Geometry check sheet. Reference: the model listing, model coordinates, mm. Face numbers are marked on the shaded views. A direction names the side the tool comes from. Coordinates: 2 decimals unless noted, no trailing zeros. Loops run counter-clockwise (first coordinate to the right, second up) from the corner with the lowest first, then second, coordinate; pieces in that order, holes last. Notation, with made-up numbers: (4.25, 15.5) -> (45.25, 15.5) arc R26 cw to (45.25, 50.5) -> close; hole circle Ø4 at (-33.5, 30). An arc over 180 degrees is marked (long way). Answer as a JSON object with one key per item and string values.
from build123d import *

# Parameters (mm, degrees)
F0_W     = 334.264
F0_H     = 232.664
F0_W_2   = 330.2
F0_H_2   = 228.6
F1_DEPTH = 53.34
F2_DEPTH = 1.27
F3_W     = 360.172
F3_H     = 258.572
F3_W_2   = 334.264
F3_H_2   = 232.664
F4_DEPTH = 2.032
F5_R     = 5.08
F6_R     = 3.175
F7_DEPTH = 1.271


with BuildPart() as f1:
    # F0 (on Top) → F1 (new body)
    with BuildSketch(Plane.XY):
        with Locations((167.132, 116.332)):
            Rectangle(F0_W, F0_H)
        with Locations((167.132, 116.332)):
            Rectangle(F0_W_2, F0_H_2, mode=Mode.SUBTRACT)
    extrude(amount=F1_DEPTH)

    # F0 (on Top) → F2 (join)
    with BuildSketch(Plane.XY):
        with Locations((167.132, 116.332)):
            Rectangle(F0_W_2, F0_H_2)
    extrude(amount=F2_DEPTH)

    # F3 (on face) → F4 (join)
    with BuildSketch(Plane.XY.offset(53.34)):
        with Locations((167.132, 116.332)):
            Rectangle(F3_W, F3_H)
        with Locations((167.132, 116.332)):
            Rectangle(F3_W_2, F3_H_2, mode=Mode.SUBTRACT)
    extrude(amount=-F4_DEPTH)

    # F5
    f5_edges = [f1.edges().sort_by_distance(p)[0] for p in [
        (334.264, 0, 25.654),
        (334.264, 232.664, 25.654),
        (0, 232.664, 25.654),
        (0, 0, 25.654),
    ]]
    fillet(f5_edges, radius=F5_R)

    # F6 (on face) → F7 (cut, through all)
    with BuildSketch(Plane.XY.offset(1.27)):
        with Locations((167.132, 116.332)):
            Circle(F6_R)
    extrude(amount=-F7_DEPTH, mode=Mode.SUBTRACT)


solid = f1.part
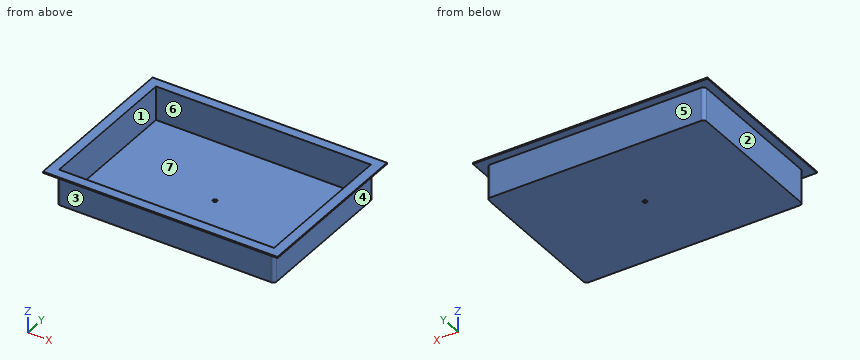
1. Section check C-C, the plane x = 78. Record the boundary of the cut face in (y, z), then the cut area to 3 significant figures.
Evaluation:
{"outline": "(-12.95, 51.31) -> (0, 51.31) -> (0, 0) -> (232.66, 0) -> (232.66, 51.31) -> (245.62, 51.31) -> (245.62, 53.34) -> (230.63, 53.34) -> (230.63, 1.27) -> (2.03, 1.27) -> (2.03, 53.34) -> (-12.95, 53.34) -> close", "area": "560 mm^2"}
2. Mould release check, pull along Y, two halves, no side actions. Record for the marked faces 4, 5, 6 and 7: released by +Y, released by -Y, zero draft, split by the parting line, or undercut.
Evaluation:
{"face 4": "zero draft", "face 5": "released by +Y", "face 6": "undercut", "face 7": "undercut"}
3. Depth check by flat-ended pin: P1, Ø3, axis at y = 65.5, z = 37.5, coming from the -X side; P2, Ø4, axis at x = 255, y = 92.5, coming from the +Z side; P3, Ø5.5, axis at x = 167.132, y = 116.332, coming from the +Z side; P4, Ø1, axis at x = 187.5, z = 25.5, coming from the -Y side. Enter the tip coordinate at first touch or a pass-through.
Evaluation:
{"P1": "stops at x = 0", "P2": "stops at z = 1.27", "P3": "passes through", "P4": "stops at y = 0"}
4. Section check B-B, the plane y = 25.5. Record the boundary of the cut face in (x, z).
Evaluation:
{"outline": "(-12.95, 51.31) -> (0, 51.31) -> (0, 0) -> (334.26, 0) -> (334.26, 51.31) -> (347.22, 51.31) -> (347.22, 53.34) -> (332.23, 53.34) -> (332.23, 1.27) -> (2.03, 1.27) -> (2.03, 53.34) -> (-12.95, 53.34) -> close"}
5. Tool access check on the marked faces 1, 2 and 3. Record the directions out of +Z, -Z, +X, -X, +Y, -Y that give a thin tool (end or side, any length) a straight path to the whole face; none if there is none.
Evaluation:
{"face 1": "+Z", "face 2": "-Z, -X, +Y, -Y", "face 3": "-Z, +X, -X, -Y"}
6. Thickness scan on probe 1 along X at (y, z) = (29.5, 49.5); probe 2 along Y at (x, z) = (285, 34); probe 3 along Z at (x, y) = (159.5, 65.5). Record the ranges inside material, lowest first. Write a range as from..to.
Evaluation:
{"probe 1": "x = 0..2.03, 332.23..334.26", "probe 2": "y = 0..2.03, 230.63..232.66", "probe 3": "z = 0..1.27"}
7. Section check A-A, the plane z = 35. Record the boundary of the cut face in (x, y).
Evaluation:
{"outline": "(0, 5.08) arc R5.08 ccw to (5.08, 0) -> (329.18, 0) arc R5.08 ccw to (334.26, 5.08) -> (334.26, 227.58) arc R5.08 ccw to (329.18, 232.66) -> (5.08, 232.66) arc R5.08 ccw to (0, 227.58) -> close; hole (2.03, 2.03) -> (332.23, 2.03) -> (332.23, 230.63) -> (2.03, 230.63) -> close"}
